Read the model definition and answer for the solid it produces. Units are mm, in the model's axes. Face numbers are marked on the shaded views. Coordinates: 2 decimals unless noted, no trailing zeros. Answer in a Markdown table with one row per item.
from build123d import *

# Parameters (mm, degrees)
F0_W     = 101.6
F0_H     = 101.6
F1_DEPTH = 50.8
F2_R     = 12.7
F3_DEPTH = 6.35


with BuildPart() as f1:
    # F0 (on Front) → F1 (new body, symmetric)
    with BuildSketch(Plane.XZ):
        Rectangle(F0_W, F0_H)
    extrude(amount=F1_DEPTH, both=True)

    # F2 (on face) → F3 (cut)
    with BuildSketch(Plane.XZ.offset(50.8)):
        with Locations((50.8, 31.75)):
            Circle(F2_R)
    extrude(amount=-F3_DEPTH, mode=Mode.SUBTRACT)


solid = f1.part
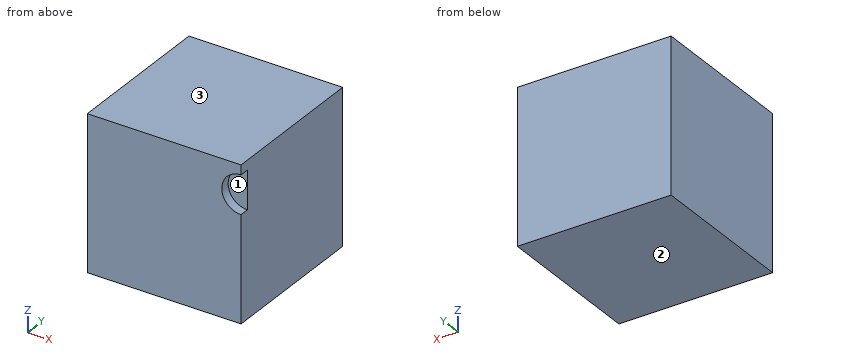
Q1. Consider line 1 (Y direction, x = 47, z = 23). Determine where the line is inside the solid, lowest interval first.
Outcome:
| item | result |
|---|---|
| line 1 | -44.45 to 50.8 |
Q2. For a pull along Z with two mould halves and no side action, classify the marked faces 1, 2 and 3 as pulls with the +Z half, pulls with the -Z half, needs draft (parallel to the pull), parting line crosses it, or undercut.
Outcome:
| item | result |
|---|---|
| face 1 | undercut |
| face 2 | pulls with the -Z half |
| face 3 | pulls with the +Z half |
Q3. Given pin 1 (6.5 mm diameter, centred on x = 46, z = 32.5, fed in from -Y), flat-ended and moving along its own axis, determine where the tip first touches the part or whether it passes through.
Outcome:
| item | result |
|---|---|
| pin 1 | y = -44.45 |
